```python
from build123d import *

# Parameters (mm, degrees)
F1_R     = 38.1
F2_DEPTH = 19.05


with BuildPart() as f2:
    # F1 (on Front) → F2 (new body)
    with BuildSketch(Plane.XZ):
        with BuildLine():
            ThreePointArc((-59.101749, 22.104146), (-11.231421, -62.092392), (63.1, 0))
            ThreePointArc((63.1, 0), (59.883643, 19.888671), (50.562465, 37.749797))
            ThreePointArc((50.562465, 37.749797), (-8.912151, 62.46746), (-59.101749, 22.104146))
        make_face()
        Circle(F1_R, mode=Mode.SUBTRACT)
        with BuildLine():
            ThreePointArc((50.562465, 37.749797), (59.883643, 19.888671), (63.1, 0))
            ThreePointArc((63.1, 0), (-11.231421, -62.092392), (-59.101749, 22.104146))
            Line((-59.101749, 22.104146), (-103.631373, -96.958523))
            Line((-103.631373, -96.958523), (-98.76699, -101.040224))
            ThreePointArc((-98.76699, -101.040224), (-64.691543, -82.67794), (-27.310033, -92.72445))
            ThreePointArc((-27.310033, -92.72445), (-25.044487, -93.333329), (-22.979308, -92.220464))
            Line((-22.979308, -92.220464), (-12.716697, -79.98996))
            Line((-12.716697, -79.98996), (286.442809, -331.014591))
            Line((286.442809, -331.014591), (290.740471, -326.339915))
            ThreePointArc((290.740471, -326.339915), (288.937178, -246.888288), (309.576211, -170.142975))
            ThreePointArc((309.576211, -170.142975), (196.952283, -176.818858), (259.002256, -82.592973))
            ThreePointArc((259.002256, -82.592973), (142.400804, -43.867073), (50.562465, 37.749797))
        make_face()
        with BuildLine():
            ThreePointArc((314.691205, -145.25625), (298.757121, -103.339829), (259.002256, -82.592973))
            ThreePointArc((259.002256, -82.592973), (196.952283, -176.818858), (309.576211, -170.142975))
            ThreePointArc((309.576211, -170.142975), (313.39923, -157.959716), (314.691205, -145.25625))
        make_face()
        with Locations((251.591205, -145.25625)):
            Circle(F1_R, mode=Mode.SUBTRACT)
    extrude(amount=F2_DEPTH)


solid = f2.part
```
Source: CAD feature listing. Evaluate the final solid. Frame: model axes, mm. A direction names the side the tool comes from. Give positions to 0.01 mm unless a question says otherwise; leave off trailing zeros. Loops run counter-clockwise (first coordinate to the right, second up) from the corner with the lowest first, then second, coordinate; pieces in that order, holes last. Notation, with made-up numbers: (81.5, 62.25) -> (103.5, 62.25) arc R14 cw to (103.5, 84.25) -> close; hole circle Ø10 at (42, -19). An arc over 180 degrees is marked (long way). Put each result on its own line as item: value. Start each with the question number.
1) Material intervals for probe 1 along Z at (x, y) = (21, -11.25); probe 2 along X at (y, z) = (-1, 7.5); probe 3 along X at (y, z) = (-4.75, 5), sorted ascending.
2) Cut plane D-D (x = 127.5). Return loops of the section in (y, z).
3) Cut plane B-B (x = 15.5). Return loops of the section in (y, z).
4) Contact query for flat-ended pins moving along their axis: P1, Ø1, axis at y = -14.5, z = -202, coming from the -X side; P2, Ø2, axis at x = 234, y = -5.5, coming from the -Z side; P3, Ø10, axis at x = 93.5, y = -3, coming from the +Z side (3 decimals); P4, Ø6, axis at x = 83, z = -9, coming from the +Y side. Output: stop coordinate, or through.
5) Reachability of faces 5 (the face through (-17.92, -9.39, -86.19)), 6 (the face through (120, 0, -118)) from +Z, -Z, +X, -X, +Y, -Y: full face, straight path, thin tool, end or side. Return the list, or none.
6) Cut plane A-A (z = -175). Return loops of the section in (x, y).
7) Cut plane C-C (y = -9). State how many separate pieces and enclosed holes the cut face has, then the cut area to 3 significant figures.
8) Draft query along Z for faces 1 (the face through (246.63, -9.39, -107.48)), 2 (the face through (288.806, -9.392, -247.997)), 3 (the face through (120, -19.05, -118)), 4 (the face through (143.903, -9.392, -44.729)). Return one class per face: released by +Z, released by -Z, zero draft, split by the parting line, or undercut.
Results are:
1. probe 1: z = -108.28 to -31.79, 31.79 to 59.5
1. probe 2: x = -64.56 to -37.35, 37.35 to 76.39
1. probe 3: x = -65.5 to -37.77, 37.77 to 78.85
2. outline: (-19.05, -197.65) -> (0, -197.65) -> (0, -34.68) -> (-19.05, -34.68) -> close
3. outline: (-19.05, -103.67) -> (0, -103.67) -> (0, -34.8) -> (-19.05, -34.8) -> close; (-19.05, 34.8) -> (0, 34.8) -> (0, 61.17) -> (-19.05, 61.17) -> close
4. P1: stops at x = 132.09
4. P2: stops at z = -287.85
4. P3: stops at z = -4.275
4. P4: stops at y = 0
5. face 5: -Z, +Y, -Y
5. face 6: +Z, -Z, +X, -X, +Y
6. outline: (100.51, -19.05) -> (227.78, -19.05) -> (227.78, 0) -> (100.51, 0) -> close; (275.4, -19.05) -> (307.55, -19.05) -> (307.55, 0) -> (275.4, 0) -> close
7. separate pieces: 1
7. enclosed holes: 2
7. area: 56,200 mm2
8. face 1: undercut
8. face 2: undercut
8. face 3: zero draft
8. face 4: released by +Z
